```python
from build123d import *

# Parameters (mm, degrees)
SKETCH2_R           = 2.35
SKETCH2_R_2         = 1.275
BOSS_EXTRUDE3_DEPTH = 0.5
SKETCH2_7_R         = 3.45
SKETCH2_7_R_2       = 2.35
BOSS_EXTRUDE5_DEPTH = 2.5
SKETCH1_R           = 2.35
SKETCH1_R_2         = 0.5
BOSS_EXTRUDE6_DEPTH = 1.5


with BuildPart() as part:
    # Sketch2 → Boss-Extrude3 (new body)
    with BuildSketch(Plane(origin=(0, 1.5, 0), x_dir=(1, 0, 0), z_dir=(0, 1, 0))):
        Circle(SKETCH2_R)
        Circle(SKETCH2_R_2, mode=Mode.SUBTRACT)
    extrude(amount=-BOSS_EXTRUDE3_DEPTH)



with BuildPart() as body_2:
    # Sketch2_7 → Boss-Extrude5 (new body)
    with BuildSketch(Plane(origin=(0, 1.5, 0), x_dir=(1, 0, 0), z_dir=(0, 1, 0))):
        Circle(SKETCH2_7_R)
        Circle(SKETCH2_7_R_2, mode=Mode.SUBTRACT)
    extrude(amount=BOSS_EXTRUDE5_DEPTH)


with BuildPart() as part_1:
    add(part.part)

    add(body_2.part)  # Boss-Extrude6 merges body 2
    # Sketch1 → Boss-Extrude6 (add)
    with BuildSketch(Plane(origin=(0, 0, 0), x_dir=(1, 0, 0), z_dir=(0, 1, 0))):
        with BuildLine():
            Line((14.35, 1.5), (1.879742768, 2.892933999))
            ThreePointArc((1.879742768, 2.892933999), (-0.020024107, 3.449941889), (-1.913197247, 2.870919068))
            Line((-1.913197247, 2.870919068), (-14.35, 1.5))
            ThreePointArc((-14.35, 1.5), (-15.85, 0), (-14.35, -1.5))
            Line((-14.35, -1.5), (-1.879742768, -2.892933999))
            ThreePointArc((-1.879742768, -2.892933999), (0.020024107, -3.449941889), (1.913197247, -2.870919068))
            Line((1.913197247, -2.870919068), (14.35, -1.5))
            ThreePointArc((14.35, -1.5), (15.85, 0), (14.35, 1.5))
        make_face()
        Circle(SKETCH1_R, mode=Mode.SUBTRACT)
        with Locations((12.35, 0)):
            Circle(SKETCH1_R_2, mode=Mode.SUBTRACT)
        with Locations((14.35, 0)):
            Circle(SKETCH1_R_2, mode=Mode.SUBTRACT)
        with Locations((10.35, 0)):
            Circle(SKETCH1_R_2, mode=Mode.SUBTRACT)
        with Locations((8.35, 0)):
            Circle(SKETCH1_R_2, mode=Mode.SUBTRACT)
        with Locations((6.35, 0)):
            Circle(SKETCH1_R_2, mode=Mode.SUBTRACT)
        with Locations((4.35, 0)):
            Circle(SKETCH1_R_2, mode=Mode.SUBTRACT)
        with Locations((-12.35, 0)):
            Circle(SKETCH1_R_2, mode=Mode.SUBTRACT)
        with Locations((-14.35, 0)):
            Circle(SKETCH1_R_2, mode=Mode.SUBTRACT)
        with Locations((-10.35, 0)):
            Circle(SKETCH1_R_2, mode=Mode.SUBTRACT)
        with Locations((-8.35, 0)):
            Circle(SKETCH1_R_2, mode=Mode.SUBTRACT)
        with Locations((-6.35, 0)):
            Circle(SKETCH1_R_2, mode=Mode.SUBTRACT)
        with Locations((-4.35, 0)):
            Circle(SKETCH1_R_2, mode=Mode.SUBTRACT)
    extrude(amount=BOSS_EXTRUDE6_DEPTH)


solid = part_1.part
```
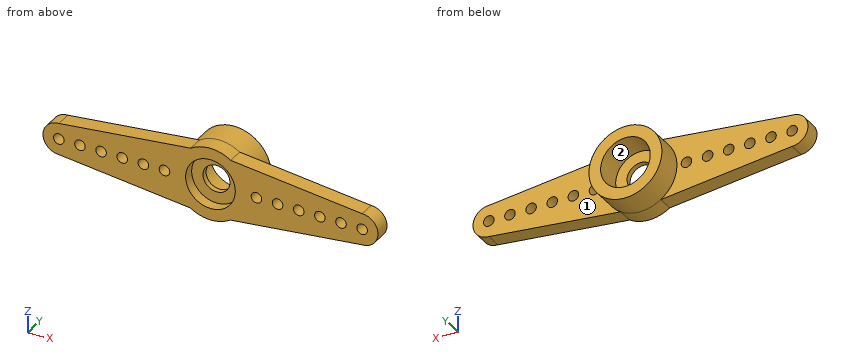
The listing builds one solid part. Answer for the finished solid, in the listing's coordinates (mm). Face numbers are marked on the shaded views. Coordinates: 2 decimals unless noted, no trailing zeros. Loops run counter-clockwise (first coordinate to the right, second up) from the corner with the lowest first, then second, coordinate; pieces in that order, holes last. Notation, with made-up numbers: (23, 51) -> (58, 51) arc R13 cw to (58, 66) -> close; hole circle Ø6 at (57, 36.5). An arc over 180 degrees is marked (long way). Return JSON: item names as keys, results as strings. Group by question number.
(1) Given pin 1 Ø3 at (x, z) = (-0.5, 0) entering from -Y; pin 2 Ø2.5 at (x, z) = (0, -0.5) entering from +Y, each flat-ended and moving along its own axis, determine where each tip first touches the part or whether it passes through.
(2) A cutting plane is placed at D-D on y = 2.45. Write down the section's boundary in (x, z).
(3) Determine the mould class of the marked faces 1 and 2 for opening direction Z: released by +Z, released by -Z, zero draft, split by the parting line, or undercut.
(4) Find the intervals of material crossed by probe 1 along Z at (x, y) = (0, 1.25) (3 decimals); probe 2 along Z at (x, y) = (-14.35, 0.8); probe 3 along Y at (x, z) = (3.5, -2.5), in increasing order. Write a range as from..to.
(5) A cutting plane is placed at A-A on x = 12.5. Write down the section's boundary in (y, z), and give its area (3 significant figures).
(6) A cutting plane is placed at B-B on y = 0.4. Count the separate pieces of the cut face and the enclosed holes in it, and give its area (3 significant figures).
The answers:
{
 "1": {"pin 1": "stops at y = 1", "pin 2": "stops at y = 1.5"},
 "2": {"outline": "circle Ø6.9 at (0, 0); hole circle Ø4.7 at (0, 0)"},
 "3": {"face 1": "zero draft", "face 2": "undercut"},
 "4": {"probe 1": "z = -3.45..-1.275, 1.275..3.45", "probe 2": "z = -1.5..-0.5, 0.5..1.5", "probe 3": "y = 0..1.5"},
 "5": {"outline": "(0, -1.71) -> (1.5, -1.71) -> (1.5, -0.48) -> (0, -0.48) -> close; (0, 0.48) -> (1.5, 0.48) -> (1.5, 1.7) -> (0, 1.7) -> close", "area": "3.68 mm^2"},
 "6": {"separate pieces": "1", "enclosed holes": "13", "area": "114 mm^2"}
}
